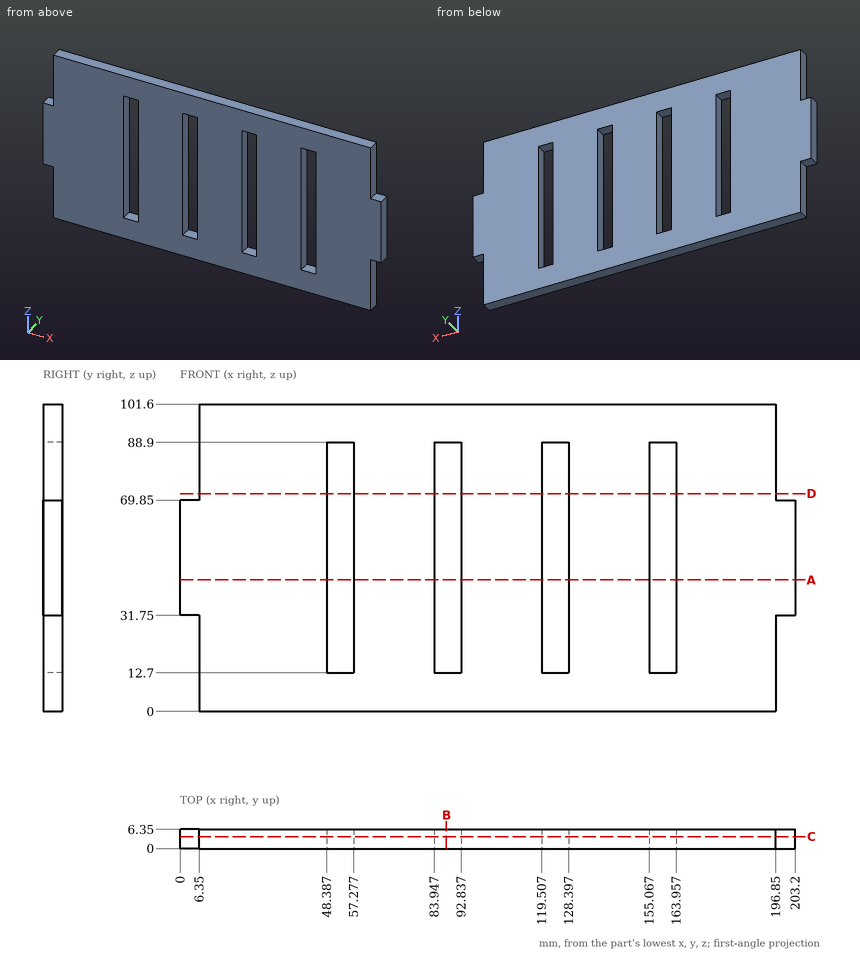
Drawing for the job (mm, zero at the part's lowest x, y, z). Give positions to 0.01 mm unless a question says otherwise; leave off trailing zeros. Write each loop counter-clockwise with the first axis right and the second up, starting at its lowest first coordinate (ties: lowest second). Pieces come first, ordered by that corner, then holes. Notation, with made-up numbers: (79, 2) -> (120, 2) arc R12 cw to (120, 20) -> close; hole circle Ø5 at (69.5, 87.5). An arc over 180 degrees is marked (long way). Put each result on its own line as item: value. Start each with the question number.
Item 1: Pin check, flat tips, straight feed: pin 1 Ø3 at (y, z) = (3, 21.5) entering from -X; pin 2 Ø3 at (y, z) = (3.5, 16.5) entering from +X; pin 3 Ø1.9 at (x, y) = (199, 3.5) entering from +Z. Stop position of each tip, or through.
Item 2: Wall check: L1, parallel to X at y = 1.5, z = 65; L2, parallel to X at y = 4.25, z = 24; L3, parallel to Z at x = 159.5, y = 5. Give the ranges that are in metal, low to high. Write a range as [from, to].
Item 3: Cut at A-A (z = 43.5). List the corners of the cut face in (x, y), then the cut area to 3 significant figures.
Item 4: Cut at D-D (z = 72). List the corners of the cut face in (x, y).
Item 5: Cut at B-B (x = 88). List the corners of the cut face in (y, z), then the cut area to 3 significant figures.
Item 6: Cut at C-C (y = 4). List the corners of the cut face in (x, z), then the cut area to 3 significant figures.
Answer list:
1. pin 1: stops at x = 6.35
1. pin 2: stops at x = 196.85
1. pin 3: stops at z = 69.85
2. L1: x = [0, 48.39], [57.28, 83.95], [92.84, 119.51], [128.4, 155.07], [163.96, 203.2]
2. L2: x = [6.35, 48.39], [57.28, 83.95], [92.84, 119.51], [128.4, 155.07], [163.96, 196.85]
2. L3: z = [0, 12.7], [88.9, 101.6]
3. outline: (0, 0) -> (48.39, 0) -> (48.39, 6.35) -> (0, 6.35) -> close; (57.28, 0) -> (83.95, 0) -> (83.95, 6.35) -> (57.28, 6.35) -> close; (92.84, 0) -> (119.51, 0) -> (119.51, 6.35) -> (92.84, 6.35) -> close; (128.4, 0) -> (155.07, 0) -> (155.07, 6.35) -> (128.4, 6.35) -> close; (163.96, 0) -> (203.2, 0) -> (203.2, 6.35) -> (163.96, 6.35) -> close
3. area: 1,060 mm2
4. outline: (6.35, 0) -> (48.39, 0) -> (48.39, 6.35) -> (6.35, 6.35) -> close; (57.28, 0) -> (83.95, 0) -> (83.95, 6.35) -> (57.28, 6.35) -> close; (92.84, 0) -> (119.51, 0) -> (119.51, 6.35) -> (92.84, 6.35) -> close; (128.4, 0) -> (155.07, 0) -> (155.07, 6.35) -> (128.4, 6.35) -> close; (163.96, 0) -> (196.85, 0) -> (196.85, 6.35) -> (163.96, 6.35) -> close
5. outline: (0, 0) -> (6.35, 0) -> (6.35, 12.7) -> (0, 12.7) -> close; (0, 88.9) -> (6.35, 88.9) -> (6.35, 101.6) -> (0, 101.6) -> close
5. area: 161 mm2
6. outline: (0, 31.75) -> (6.35, 31.75) -> (6.35, 0) -> (196.85, 0) -> (196.85, 31.75) -> (203.2, 31.75) -> (203.2, 69.85) -> (196.85, 69.85) -> (196.85, 101.6) -> (6.35, 101.6) -> (6.35, 69.85) -> (0, 69.85) -> close; hole (48.39, 12.7) -> (57.28, 12.7) -> (57.28, 88.9) -> (48.39, 88.9) -> close; hole (83.95, 12.7) -> (92.84, 12.7) -> (92.84, 88.9) -> (83.95, 88.9) -> close; hole (119.51, 12.7) -> (128.4, 12.7) -> (128.4, 88.9) -> (119.51, 88.9) -> close; hole (155.07, 12.7) -> (163.96, 12.7) -> (163.96, 88.9) -> (155.07, 88.9) -> close
6. area: 17,100 mm2
